```python
from build123d import *

# Parameters (mm, degrees)
SKETCH1_W           = 55
SKETCH1_H           = 70
BOSS_EXTRUDE1_DEPTH = 3
SKETCH2_R           = 1.5
CUT_EXTRUDE1_DEPTH  = 3
FILLET1_R           = 5


with BuildPart() as part:
    # Sketch1 → Boss-Extrude1 (new body)
    with BuildSketch(Plane.XY):
        with Locations((1.762820513, 7.248931624)):
            Rectangle(SKETCH1_W, SKETCH1_H)
    extrude(amount=BOSS_EXTRUDE1_DEPTH)

    # Sketch2 → Cut-Extrude1 (cut)
    with BuildSketch(Plane.XY.offset(3)):
        with Locations((-20.737179487, 36.587967336)):
            Circle(SKETCH2_R)
        with Locations((24.262820513, 36.587967336)):
            Circle(SKETCH2_R)
        with Locations((-20.737179487, 18.087967336)):
            Circle(SKETCH2_R)
        with Locations((24.262820513, 18.087967336)):
            Circle(SKETCH2_R)
        with Locations((-20.737179487, -22.751068376)):
            Circle(SKETCH2_R)
        with Locations((24.262820513, -22.751068376)):
            Circle(SKETCH2_R)
    extrude(amount=-CUT_EXTRUDE1_DEPTH, mode=Mode.SUBTRACT)

    # Fillet1
    fillet1_edges = [part.edges().sort_by_distance(p)[0] for p in [
        (-25.737179487, 42.248931624, 1.5),
        (29.262820513, 42.248931624, 1.5),
        (29.262820513, -27.751068376, 1.5),
        (-25.737179487, -27.751068376, 1.5),
    ]]
    fillet(fillet1_edges, radius=FILLET1_R)


solid = part.part
```
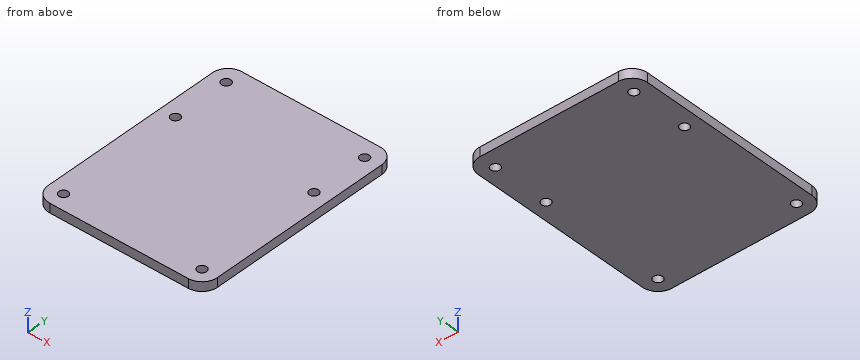
The model under review builds one solid part; all positions refer to its coordinate system, in mm. Round coordinates to 2 decimals unless told otherwise and drop trailing zeros. Loops run counter-clockwise (first coordinate to the right, second up) from the corner with the lowest first, then second, coordinate; pieces in that order, holes last. Notation, with made-up numbers: (-9, -34.75) -> (21, -34.75) arc R20 cw to (21, -7.75) -> close; hole circle Ø9 at (-23.75, 52.25). An arc over 180 degrees is marked (long way). Answer in a Markdown table with one row per item.
1) Wall thickness on line 1 along Y through (x, z) = (-20, 2.75); line 2 along X through (y, z) = (-23, 0.5); line 3 along Y through (x, z) = (-22.5, 0.2): over which ranges is each line inside the solid? List them lowest first.
Taken from the geometry:
| item | result |
|---|---|
| line 1 | y = -27.75 to -24.06, -21.44 to 16.78, 19.39 to 35.28, 37.89 to 42.25 |
| line 2 | x = -25.73 to -22.22, -19.26 to 22.78, 25.74 to 29.26 |
| line 3 | y = -27.43 to 41.93 |
2) For pin 1 Ø2.5 at (x, y) = (-20.74, 36.59) entering from +Z, flat-tipped, find the tip position at first contact; note if it passes through.
Taken from the geometry:
| item | result |
|---|---|
| pin 1 | passes through |
3) Consider section A-A, the plane z = 1.25. Write out the cut boundary in (x, y).
Taken from the geometry:
| item | result |
|---|---|
| outline | (-25.74, -22.75) arc R5 ccw to (-20.74, -27.75) -> (24.26, -27.75) arc R5 ccw to (29.26, -22.75) -> (29.26, 37.25) arc R5 ccw to (24.26, 42.25) -> (-20.74, 42.25) arc R5 ccw to (-25.74, 37.25) -> close; hole circle Ø3 at (-20.74, -22.75); hole circle Ø3 at (-20.74, 18.09); hole circle Ø3 at (-20.74, 36.59); hole circle Ø3 at (24.26, -22.75); hole circle Ø3 at (24.26, 18.09); hole circle Ø3 at (24.26, 36.59) |
